Can you work these out from the model? Positions are in its coordinate system, mm. Face numbers are marked on the shaded views. A direction names the side the tool comes from. Coordinates: 2 decimals unless noted, no trailing zeros. Write each loop counter-clockwise with the first axis right and the second up, starting at its lowest first coordinate (ties: lowest second). Pieces come first, ordered by that corner, then holes. Notation, with made-up numbers: (9.5, -39.5) -> (33.5, -39.5) arc R16 cw to (33.5, -20.5) -> close; hole circle Ø1 at (-15.75, 6). An arc over 180 degrees is marked (long way). Use one line per item in the form item = value.
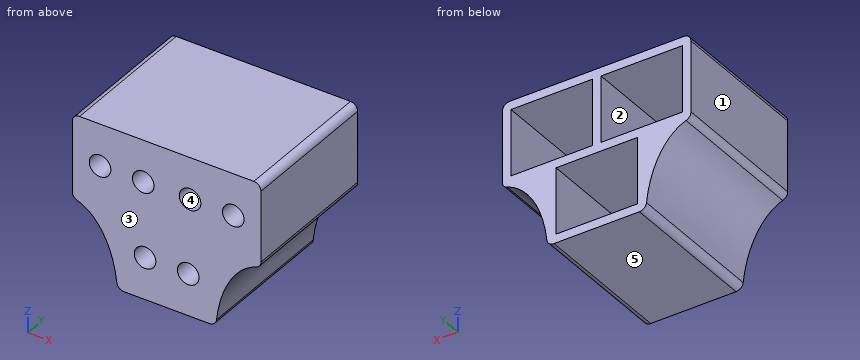
```python
from build123d import *

# Parameters (mm, degrees)
SKETCH1_W               = 13.1
SKETCH1_H               = 5.8
BOSS_EXTRUDE1_DEPTH     = 5
SKETCH10_W              = 5.65
SKETCH10_H              = 4.6
CUT_EXTRUDE7_DEPTH      = 6.6
CUT_EXTRUDE6_DEPTH      = 9.735702605
CUT_EXTRUDE6_DEPTH_BACK = 9.735702605
SKETCH9_R               = 0.75
BOSS_EXTRUDE2_START     = -5
BOSS_EXTRUDE2_DEPTH     = 10
SKETCH12_W              = 5.65
SKETCH12_H              = 4.6
SKETCH12_R              = 0.75
BOSS_EXTRUDE3_DEPTH     = 3.4
FILLET1_START           = -5
FILLET1_DEPTH           = 10
FILLET2_R               = 0.5


with BuildPart() as part:
    # Sketch1 → Boss-Extrude1 (new, symmetric)
    with BuildSketch(Plane(origin=(0, 0, 0), x_dir=(1, 0, 0), z_dir=(0, 1, 0))):
        Rectangle(SKETCH1_W, SKETCH1_H)
    extrude(amount=BOSS_EXTRUDE1_DEPTH, both=True)

    # Sketch10 → Cut-Extrude7 (cut)
    with BuildSketch(Plane(origin=(0, 5, 0), x_dir=(1, 0, 0), z_dir=(0, 1, 0))):
        with Locations((-3.125, 0)):
            Rectangle(SKETCH10_W, SKETCH10_H)
        with Locations((3.125, 0)):
            Rectangle(SKETCH10_W, SKETCH10_H)
    extrude(amount=-CUT_EXTRUDE7_DEPTH, mode=Mode.SUBTRACT)

    # Sketch9 → Cut-Extrude6 (cut, two sides: drawn at the far end of the back side and taken through both)
    with BuildSketch(Plane(origin=(0, 0, 0), x_dir=(1, 0, 0), z_dir=(0, 1, 0)).offset(-CUT_EXTRUDE6_DEPTH_BACK)):
        with Locations(Location((-4.625, 0, 0), (0, 0, 270))):
            Circle(SKETCH9_R)
        with Locations(Location((-1.625, 0, 0), (0, 0, 270))):
            Circle(SKETCH9_R)
        with Locations(Location((1.625, 0, 0), (0, 0, 270))):
            Circle(SKETCH9_R)
        with Locations(Location((4.625, 0, 0), (0, 0, 270))):
            Circle(SKETCH9_R)
    extrude(amount=CUT_EXTRUDE6_DEPTH + CUT_EXTRUDE6_DEPTH_BACK, mode=Mode.SUBTRACT)

    # Sketch11 → Boss-Extrude2 (add)
    with BuildSketch(Plane(origin=(0, 0, 0), x_dir=(1, 0, 0), z_dir=(0, 1, 0)).offset(BOSS_EXTRUDE2_START)):
        Polygon((-3.425, 8.1), (-3.425, 2.9), (-2.825, 2.9), (-2.825, 7.5), (2.825, 7.5), (2.825, 2.9), (3.425, 2.9), (3.425, 8.1), align=None)
    extrude(amount=BOSS_EXTRUDE2_DEPTH)

    # Sketch12 → Boss-Extrude3 (add)
    with BuildSketch(Plane.XZ.offset(5)):
        with Locations((0, -5.2)):
            Rectangle(SKETCH12_W, SKETCH12_H)
        with Locations(Location((-1.5, -5.2, 0), (0, 0, 270))):
            Circle(SKETCH12_R, mode=Mode.SUBTRACT)
        with Locations(Location((1.5, -5.2, 0), (0, 0, 270))):
            Circle(SKETCH12_R, mode=Mode.SUBTRACT)
    extrude(amount=-BOSS_EXTRUDE3_DEPTH)

    # Fillet1: read off the stored shape, not the designer's step
    # Fillet1 outline → Fillet1 (add)
    with BuildSketch(Plane(origin=(0, 0, 0), x_dir=(1, 0, 0), z_dir=(0, 1, 0)).offset(FILLET1_START)):
        with BuildLine():
            add(Edge.make_bspline(
                [(3.425, 8.1), (3.699466412, 3.355749046), (6.55, 2.9)],
                knots=[0, 0, 0, 1, 1, 1], degree=2, weights=[1, 0.779308952, 1]))
            Line((3.425, 8.1), (3.425, 2.9))
            Line((3.425, 2.9), (6.55, 2.9))
        make_face()
        with BuildLine():
            Line((-3.425, 2.9), (-3.425, 8.1))
            add(Edge.make_bspline(
                [(-3.425, 8.1), (-3.699466412, 3.355749046), (-6.55, 2.9)],
                knots=[0, 0, 0, 1, 1, 1], degree=2, weights=[1, 0.779308952, 1]))
            Line((-6.55, 2.9), (-3.425, 2.9))
        make_face()
    extrude(amount=FILLET1_DEPTH)

    # Fillet2
    fillet2_edges = [part.edges().sort_by_distance(p)[0] for p in [
        (-6.55, 0, -2.9),
        (-3.425, 0, -8.1),
        (3.425, 0, -8.1),
        (6.55, 0, -2.9),
        (6.55, 0, 2.9),
        (-6.55, 0, 2.9),
    ]]
    fillet(fillet2_edges, radius=FILLET2_R)


solid = part.part
```
Q1. Suppose I cut it at B-B (z = 1.25). Write out the boundary of the cut face in (x, y).
Return value:
outline = (-6.55, -5) -> (6.55, -5) -> (6.55, 5) -> (5.95, 5) -> (5.95, -1.6) -> (0.3, -1.6) -> (0.3, 5) -> (-0.3, 5) -> (-0.3, -1.6) -> (-5.95, -1.6) -> (-5.95, 5) -> (-6.55, 5) -> close
Q2. For the marked faces 1 and 2, which set-ups out of +Z, -Z, +X, -X, +Y, -Y let a thin tool reach every point of the face, with its end or its side?
Return value:
face_1 = +Z, -Z, -X, +Y, -Y
face_2 = +Y
Q3. If I drill on line 1 (X direction, y = 2.5, z = -0.75); line 2 (X direction, y = -4.1, z = 0) (3 decimals); line 3 (Z direction, x = -1.75, y = 1.25), over which ranges is the centre line in solid material (lowest first)? Write a range as from..to.
Return value:
line_1 = -6.55..-5.95, -0.3..0.3, 5.95..6.55
line_2 = -6.55..-5.375, -3.875..-2.375, -0.875..0.875, 2.375..3.875, 5.375..6.55
line_3 = -8.1..-7.5, -2.9..-2.3, 2.3..2.9
Q4. Suppose I cut it at C-C (y = 3.25). Give the number of separate pieces and of enclosed holes in the cut face, then the cut area to 3 significant figures.
Return value:
separate_pieces = 1
enclosed_holes = 3
area = 41.6 mm2
Q5. Thinking about a two-plate mould opening in Z: for the marked faces 3, 4 and 5, which applies, released by +Z, released by -Z, zero draft, split by the parting line, or undercut?
Return value:
face_3 = zero draft
face_4 = undercut
face_5 = released by -Z
Q6. Suppose I cut it at A-A (z = 0). Write out the boundary of the cut face in (x, y) (3 decimals), then the cut area to 3 significant figures.
Return value:
outline = (-6.55, -5) -> (-5.375, -5) -> (-5.375, -1.6) -> (-5.95, -1.6) -> (-5.95, 5) -> (-6.55, 5) -> close; (-3.875, -5) -> (-2.375, -5) -> (-2.375, -1.6) -> (-3.875, -1.6) -> close; (-0.875, -5) -> (0.875, -5) -> (0.875, -1.6) -> (0.3, -1.6) -> (0.3, 5) -> (-0.3, 5) -> (-0.3, -1.6) -> (-0.875, -1.6) -> close; (2.375, -5) -> (3.875, -5) -> (3.875, -1.6) -> (2.375, -1.6) -> close; (5.375, -5) -> (6.55, -5) -> (6.55, 5) -> (5.95, 5) -> (5.95, -1.6) -> (5.375, -1.6) -> close
area = 36.0 mm2
Q7. Will these pins go through, and if not, where does the flat tip stop? pin 1 (1.4 mm diameter, centred on y = 3, z = -6, fed in from -X); pin 2 (2.5 mm diameter, centred on x = -1.5, z = -5.2, fed in from +Y).
Return value:
pin_1 = -4.05
pin_2 = -1.6
